from build123d import *

# Parameters (mm, degrees)
F2_DEPTH = 4.001
F3_R     = 3
F4_R     = 1


with BuildPart() as f1:
    # F0 (on Right) → F1 (revolve)
    with BuildSketch(Plane.YZ):
        with BuildLine():
            Line((0, 39), (0, 0))
            Line((0, 0), (4, 0))
            Line((4, 0), (4, 16.15))
            Line((4, 16.15), (72, 16.15))
            Line((72, 16.15), (72, 23.1103692204))
            Line((72, 23.1103692204), (68, 23.1103692204))
            Line((68, 23.1103692204), (68, 27))
            Line((68, 27), (4, 27))
            Line((4, 27), (4, 39))
            ThreePointArc((4, 39), (3.7071067812, 39.7071067812), (3, 40))
            Line((3, 40), (1, 40))
            ThreePointArc((1, 40), (0.2928932188, 39.7071067812), (0, 39))
        make_face()
    revolve(axis=Axis((0, 36, 0), (0, 1, 0)))

    # F2 (cut, through all): a face of the model
    f2_faces = [f1.faces().sort_by_distance(p)[0] for p in [
        (0, 4, 0),
    ]]
    extrude(f2_faces, amount=-F2_DEPTH, mode=Mode.SUBTRACT)

    # F3
    f3_edges = [f1.edges().sort_by_distance(p)[0] for p in [
        (0, 0, -16.15),
    ]]
    fillet(f3_edges, radius=F3_R)

    # F4
    f4_edges = [f1.edges().sort_by_distance(p)[0] for p in [
        (0, 72, -23.110369),
    ]]
    fillet(f4_edges, radius=F4_R)


solid = f1.part
Work out the finished part from the listing and answer in its coordinate system (mm). A direction names the side the tool comes from. Coordinates: 2 decimals unless noted, no trailing zeros. Loops run counter-clockwise (first coordinate to the right, second up) from the corner with the lowest first, then second, coordinate; pieces in that order, holes last. Notation, with made-up numbers: (-2, 44.5) -> (6, 44.5) arc R16 cw to (6, 68.5) -> close; hole circle Ø2 at (-5.75, -37). An arc over 180 degrees is marked (long way). Write each question's results on one line, items separated by ' | '. Start each with the question number.
1) The mould has two halves that part along Z. Classify faces 3 (the flat face through (-16.3, 72, -1.5)), 4 (the cylindrical face through (-15.766, 37.983, -3.501)), 5 (the cylindrical face through (-26.36, 35.55, -5.85)): pulls with the +Z half, pulls with the -Z half, needs draft (parallel to the pull), parting line crosses it, or undercut.
2) For faces 1 (the cylindrical face through (-20.503, 69.479, 10.664)), 2 (the flat face through (18, 0, 8)), determine the directions among +Z, -Z, +X, -X, +Y, -Y from which every point of the face is accessible in a straight line to the end or side of a thin tool.
3) Flat-ended cylindrical pins translate along their axes: P1, Ø10, axis at x = -22.5, y = 55.5, coming from the +Z side; P2, Ø1.5, axis at y = 39, z = -18, coming from the -X side; P3, Ø5, axis at y = 10.5, z = 27.5, coming from the -X side; P4, Ø19.5, axis at x = 0, z = 0, coming from the +Y side. Find the tip coordinate at first contact, or state that the pin passes through.
4) Find section A-A on x = 0. Determine the outline of the cut face in (y, z).
5) Find section B-B on z = 0. Determine the outline of the cut face in (x, y), then the cut area to 3 significant figures.
6) Consider line 1 along X through (y, z) = (36, 0); line 2 along X through (y, z) = (27, 7.5); line 3 along Y through (x, z) = (-31, -0.5). Determine where each line is inside the solid, lowest interval first.
7) Find section C-C on y = 30. Determine the outline of the cut face in (x, z), then the cut area to 3 significant figures.
Response values:
1) face 3: needs draft | face 4: undercut | face 5: parting line crosses it
2) face 1: +Y | face 2: +Z, -Z, +X, -X, -Y
3) P1: stops at z = 20.56 | P2: stops at x = -20.77 | P3: stops at x = -10.2 | P4: passes through
4) outline: (0, -39) arc R1 ccw to (1, -40) -> (3, -40) arc R1 ccw to (4, -39) -> (4, -27) -> (68, -27) -> (68, -23.11) -> (71, -23.11) arc R1 ccw to (72, -22.11) -> (72, -16.15) -> (3, -16.15) arc R3 ccw to (0, -19.15) -> close; (0, 19.15) arc R3 ccw to (3, 16.15) -> (72, 16.15) -> (72, 22.11) arc R1 ccw to (71, 23.11) -> (68, 23.11) -> (68, 27) -> (4, 27) -> (4, 39) arc R1 ccw to (3, 40) -> (1, 40) arc R1 ccw to (0, 39) -> close
5) outline: (-40, 1) arc R1 ccw to (-39, 0) -> (-19.15, 0) arc R3 ccw to (-16.15, 3) -> (-16.15, 72) -> (-22.11, 72) arc R1 ccw to (-23.11, 71) -> (-23.11, 68) -> (-27, 68) -> (-27, 4) -> (-39, 4) arc R1 ccw to (-40, 3) -> close; (16.15, 3) arc R3 ccw to (19.15, 0) -> (39, 0) arc R1 ccw to (40, 1) -> (40, 3) arc R1 ccw to (39, 4) -> (27, 4) -> (27, 68) -> (23.11, 68) -> (23.11, 71) arc R1 ccw to (22.11, 72) -> (16.15, 72) -> close | area: 1,630 mm^2
6) line 1: x = -27 to -16.15, 16.15 to 27 | line 2: x = -25.94 to -14.3, 14.3 to 25.94 | line 3: y = 0 to 4
7) outline: circle Ø54 at (0, 0); hole circle Ø32.3 at (0, 0) | area: 1,470 mm^2
